Answer from the drawing. Dimensions are ordinates in mm from the lowest x, y and z of the part. Round coordinates to 2 decimals unless told otherwise and drop trailing zeros. Loops run counter-clockwise (first coordinate to the right, second up) from the corner with the lowest first, then second, coordinate; pieces in that order, holes last. Notation, with made-up numbers: (-40, -7.5) - (-17, -7.5) arc R28 cw to (-17, 17.5) - close; hole circle Ø8 at (29, 65). An arc over 180 degrees is marked (long way). Return JSON: item names as keys, results as strings.
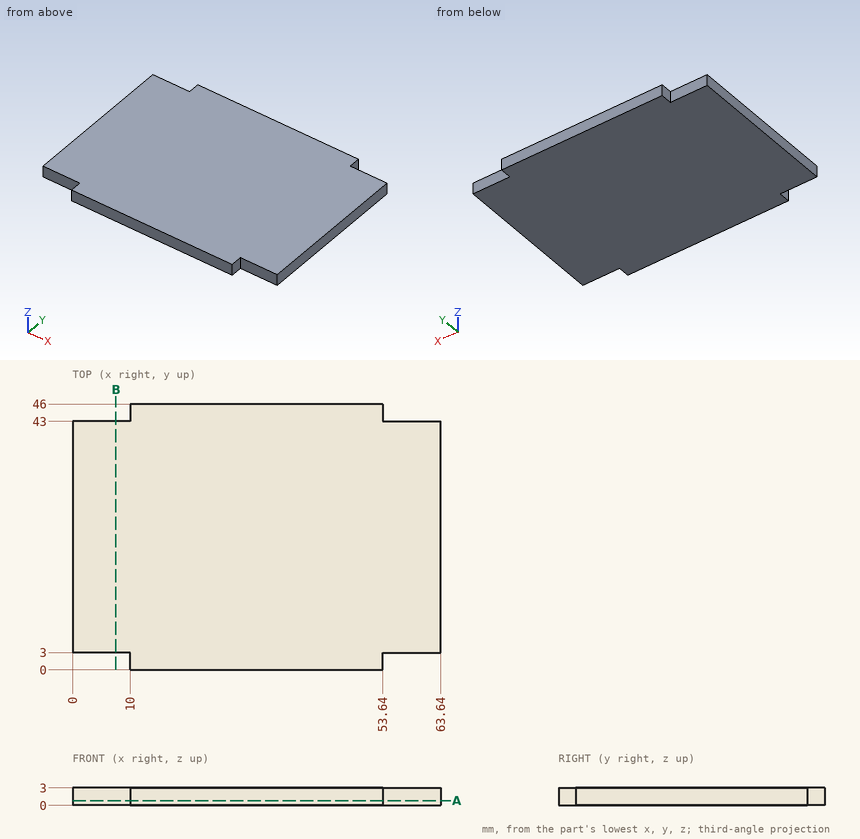
1) Section B-B (x = 7.5) is taken. Give the vertices of the cut face in (y, z), and give its area (3 significant figures).
Verdict:
{"outline": "(3, 0) - (43, 0) - (43, 3) - (3, 3) - close", "area": "120 mm2"}
2) Find the intervals of material crossed by L1, parallel to Y at x = 60, z = 1.25, in increasing order.
Verdict:
{"L1": "y = 3 to 43"}
3) Section A-A (z = 0.8) is taken. Give the vertices of the cut face in (x, y).
Verdict:
{"outline": "(0, 3) - (10, 3) - (10, 0) - (53.64, 0) - (53.64, 3) - (63.64, 3) - (63.64, 43) - (53.64, 43) - (53.64, 46) - (10, 46) - (10, 43) - (0, 43) - close"}
4) Flat-ended cylindrical pins translate along their axes: pin 1 (0.9 mm diameter, centred on y = 1.5, z = 1.5, fed in from +X); pin 2 (1.5 mm diameter, centred on x = 4, z = 1, fed in from -Y); pin 3 (0.9 mm diameter, centred on x = 6.5, z = 1, fed in from +Y). Find the tip coordinate at first contact, or state that the pin passes through.
Verdict:
{"pin 1": "stops at x = 53.64", "pin 2": "stops at y = 3", "pin 3": "stops at y = 43"}
